Input: part model. Units: mm. Frame: model coordinates. A direction names the side the tool comes from. Coordinates: 2 decimals unless noted, no trailing zeros. Order: outer loops, then holes, each group sorted by start corner. A loop starts at its lowest first (then second) coordinate and runs counter-clockwise, first axis right, second up. Notation, with made-up numbers: (73.5, -24) - (101.5, -24) arc R9 ccw to (101.5, -16) - close; hole circle Ø1 at (1, 35). An arc over 180 degrees is marked (long way). One line per question, with ' | ' between items.
from build123d import *

# Parameters (mm, degrees)
SKETCH1_W             = 8.098713366
SKETCH1_H             = 21.564091284
BOSS_EXTRUDE2_DEPTH   = 95
BOSS_EXTRUDE2_2_DEPTH = 95
SKETCH1_5_W           = 160
SKETCH1_5_H           = 80
SKETCH1_5_W_2         = 8.098713366
SKETCH1_5_H_2         = 21.564091284
BOSS_EXTRUDE3_DEPTH   = 10
SKETCH3_R             = 4.973174901
CUT_EXTRUDE1_DEPTH    = 155.631415981


with BuildPart() as part:
    # Sketch1 → Boss-Extrude2 (new body)
    with BuildSketch(Plane(origin=(0, 0, 0), x_dir=(1, 0, 0), z_dir=(0, 1, 0))):
        with Locations((-70.582059298, 0)):
            Rectangle(SKETCH1_W, SKETCH1_H)
    extrude(amount=BOSS_EXTRUDE2_DEPTH)



with BuildPart() as body_2:
    # Sketch1 → Boss-Extrude2 2 (new body)
    with BuildSketch(Plane(origin=(0, 0, 0), x_dir=(1, 0, 0), z_dir=(0, 1, 0))):
        with Locations((70.582059298, 0)):
            Rectangle(SKETCH1_W, SKETCH1_H)
    extrude(amount=BOSS_EXTRUDE2_2_DEPTH)


with BuildPart() as part_1:
    add(part.part)

    add(body_2.part)  # Boss-Extrude3 merges body 2
    # Sketch1<5> → Boss-Extrude3 (add)
    with BuildSketch(Plane(origin=(0, 0, 0), x_dir=(1, 0, 0), z_dir=(0, 1, 0))):
        Rectangle(SKETCH1_5_W, SKETCH1_5_H)
        with Locations((-70.582059298, 0)):
            Rectangle(SKETCH1_5_W_2, SKETCH1_5_H_2, mode=Mode.SUBTRACT)
        with Locations((70.582059298, 0)):
            Rectangle(SKETCH1_5_W_2, SKETCH1_5_H_2, mode=Mode.SUBTRACT)
    extrude(amount=BOSS_EXTRUDE3_DEPTH)

    # Sketch3 → Cut-Extrude1 (cut, through all)
    with BuildSketch(Plane(origin=(74.631415981, 0, 0), x_dir=(0, 0, -1), z_dir=(1, 0, 0))):
        with Locations((0, 85)):
            Circle(SKETCH3_R)
    extrude(amount=-CUT_EXTRUDE1_DEPTH, mode=Mode.SUBTRACT)


solid = part_1.part
Item 1: Section A-A on z = 0. Return the cut outline in (x, y), and give its area (3 significant figures).
Data:
outline: (-80, 0) - (80, 0) - (80, 10) - (74.63, 10) - (74.63, 80.03) - (66.53, 80.03) - (66.53, 10) - (-66.53, 10) - (-66.53, 80.03) - (-74.63, 80.03) - (-74.63, 10) - (-80, 10) - close; (-74.63, 89.97) - (-66.53, 89.97) - (-66.53, 95) - (-74.63, 95) - close; (66.53, 89.97) - (74.63, 89.97) - (74.63, 95) - (66.53, 95) - close | area: 2,820 mm^2
Item 2: Ray query, line 1 (X direction, y = 81.5, z = 6); line 2 (Y direction, x = -68, z = 0); line 3 (Y direction, x = -44, z = -35). Return the intervals inside material, ascending.
Data:
line 1: -74.63 to -66.53, 66.53 to 74.63 | line 2: 0 to 80.03, 89.97 to 95 | line 3: 0 to 10
Item 3: Section D-D on z = -17.5. Return the cut outline in (x, y), and give its area (3 significant figures).
Data:
outline: (-80, 0) - (80, 0) - (80, 10) - (-80, 10) - close | area: 1,600 mm^2
Item 4: Section B-B on x = -70. Return the cut outline in (y, z), and give its area (3 significant figures).
Data:
outline: (0, -40) - (10, -40) - (10, -10.78) - (95, -10.78) - (95, 10.78) - (10, 10.78) - (10, 40) - (0, 40) - close; hole circle Ø9.95 at (85, 0) | area: 2,560 mm^2
Item 5: Contact query for flat-ended pins moving along their axis: P1, Ø10, axis at x = -46.5, z = -28.5, coming from the +Y side; P2, Ø4, axis at x = 69, y = 36.5, coming from the +Z side; P3, Ø13, axis at y = 85, z = 0, coming from the +X side. Output: stop coordinate, or through.
Data:
P1: y = 10 | P2: z = 10.78 | P3: x = 74.63
Item 6: Draft query along X for faces 1 (the face through (-71, 52, 10.782)), 2 (the face through (-74.631, 52, 0)), 3 (the face through (74.631, 52, 0)), 4 (the face through (-66.533, 52, 0)). Return one class per face: released by +X, released by -X, zero draft, split by the parting line, or undercut.
Data:
face 1: zero draft | face 2: released by -X | face 3: released by +X | face 4: undercut
Item 7: Access query for faces 5 (the face through (-71, 95, 0)), 6 (the face through (66.533, 52, 0)), 7 (the face through (71, 52, -10.782)), 8 (the face through (71, 52, 10.782)). Directions: +Z, -Z, +X, -X, +Y, -Y. A direction counts if a zero-diameter tool reaches every point of the face in a straight line with its end or side. Return the directions, or none.
Data:
face 5: +Z, -Z, +X, -X, +Y | face 6: +Z, -Z, +Y | face 7: -Z, +X, -X, +Y | face 8: +Z, +X, -X, +Y
Item 8: Section C-C on y = 85. Return the cut outline in (x, z).
Data:
outline: (-74.63, -10.78) - (-66.53, -10.78) - (-66.53, -4.97) - (-74.63, -4.97) - close; (-74.63, 4.97) - (-66.53, 4.97) - (-66.53, 10.78) - (-74.63, 10.78) - close; (66.53, -10.78) - (74.63, -10.78) - (74.63, -4.97) - (66.53, -4.97) - close; (66.53, 4.97) - (74.63, 4.97) - (74.63, 10.78) - (66.53, 10.78) - close
